Could you check a few things on this model? Use its own coordinates, in mm. Face numbers are marked on the shaded views. Give positions to 0.01 mm unless a question says otherwise; leave off trailing zeros. Write each loop counter-clockwise with the first axis right and the second up, starting at its lowest first coordinate (ties: lowest second). Pieces come first, ordered by that corner, then holes. Notation, with made-up numbers: M -6,15.5 L 21,15.5 A19 cw 21,27.5 Z; hole C 66.5,11 d1. An arc over 180 degrees is marked long. One line per item, written item: value.
```python
from build123d import *

# Parameters (mm, degrees)
F1_DEPTH   = 18
F5_D       = 8.8
F5_ON_F4_D = 8.8
F5_ON_F3_D = 8.8


with BuildPart() as f1:
    # F0 (on Front) → F1 (new body, symmetric)
    with BuildSketch(Plane.XZ):
        Polygon((94, -63), (94, 63), (-94, 63), (-94, -63), (-114, -63), (-114, -65), (-92, -65), (-92, 61), (92, 61), (92, -65), (114, -65), (114, -63), align=None)
    extrude(amount=F1_DEPTH, both=True)

    # F5 (through all)
    with Locations(Plane.XY.offset(63)):
        with Locations((-32.5, 0), (32.5, 0)):
            Hole(F5_D / 2)

    # F5 on F4 (through all)
    with Locations(Plane.XY.offset(-63)):
        with Locations((104, 0)):
            Hole(F5_ON_F4_D / 2)

    # F5 on F3 (through all)
    with Locations(Plane.XY.offset(-63)):
        with Locations((-104, 0)):
            Hole(F5_ON_F3_D / 2)


solid = f1.part
```
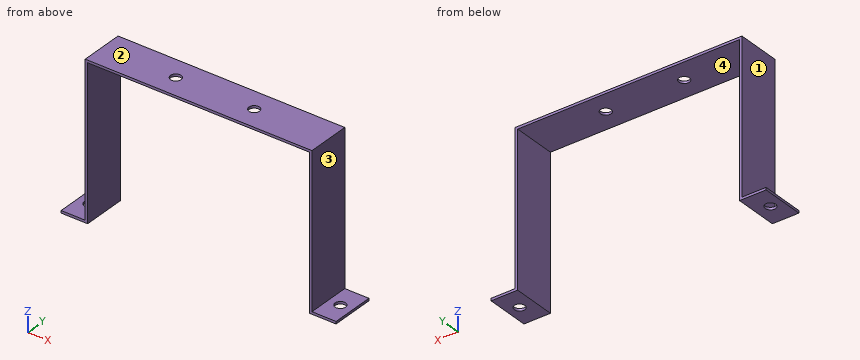
1) Please list where these lines run through material, in increasing order: L1, parallel to X at y = -0.5, z = -60; L2, parallel to Y at x = 104, z = -64; L3, parallel to Z at x = -96.5, y = -10.5. Write a range as from..to.
Outcome:
L1: x = -94..-92, 92..94
L2: y = -18..-4.4, 4.4..18
L3: z = -65..-63
2) We'd pull the mould along X, two halves only. Please class the marked faces 1, 2, 3 and 4: pulls with the +X half, pulls with the -X half, needs draft (parallel to the pull), parting line crosses it, or undercut.
Outcome:
face 1: pulls with the -X half
face 2: needs draft
face 3: pulls with the +X half
face 4: undercut
3) If we section it at D-D, the plane y = -11.5: Write out the boundary of the cut face in (x, z), then the cut area to 3 significant figures.
Outcome:
outline: M -114,-65 L -92,-65 L -92,61 L 92,61 L 92,-65 L 114,-65 L 114,-63 L 94,-63 L 94,63 L -94,63 L -94,-63 L -114,-63 Z
area: 960 mm^2
4) If we section it at A-A, the plane z = 3: Write out the boundary of the cut face in (x, y), then the cut area to 3 significant figures.
Outcome:
outline: M -94,-18 L -92,-18 L -92,18 L -94,18 Z; M 92,-18 L 94,-18 L 94,18 L 92,18 Z
area: 144 mm^2
5) If we section it at B-B, the plane y = 0: Write out the boundary of the cut face in (x, z), then the cut area to 3 significant figures.
Outcome:
outline: M -114,-65 L -108.4,-65 L -108.4,-63 L -114,-63 Z; M -99.6,-65 L -92,-65 L -92,61 L -36.9,61 L -36.9,63 L -94,63 L -94,-63 L -99.6,-63 Z; M -28.1,61 L 28.1,61 L 28.1,63 L -28.1,63 Z; M 36.9,61 L 92,61 L 92,-65 L 99.6,-65 L 99.6,-63 L 94,-63 L 94,63 L 36.9,63 Z; M 108.4,-65 L 114,-65 L 114,-63 L 108.4,-63 Z
area: 890 mm^2
6) If we section it at C-C, the plane x = 32.5: Write out the boundary of the cut face in (y, z).
Outcome:
outline: M -18,61 L -4.4,61 L -4.4,63 L -18,63 Z; M 4.4,61 L 18,61 L 18,63 L 4.4,63 Z
7) I'm going to push flat-ended pins straight in: pin 1 (2 mm diameter, centred on x = -59.5, y = 9.5, fed in from -Z); pin 2 (2 mm diameter, centred on y = -7.5, z = -9.5, fed in from -X); pin 3 (16 mm diameter, centred on x = -105, y = -0.5, fed in from +Z). Where does each tip first touch, or does it pass through?
Outcome:
pin 1: stops at z = 61
pin 2: stops at x = -94
pin 3: stops at z = -63
